```python
from build123d import *

# Parameters (mm, degrees)
SKETCH1_W               = 2000
SKETCH1_H               = 420
SKETCH1_W_2             = 1782.939992392
SKETCH1_H_2             = 340
BOSS_EXTRUDE1_DEPTH     = 20
SKETCH3_W               = 30
SKETCH3_H               = 80
BOSS_EXTRUDE2_DEPTH     = 200
FILLET1_R               = 40
FILLET2_R               = 40
SKETCH5_W               = 972.378142936
SKETCH5_H               = 20.021799472
SKETCH5_W_2             = 1944.756285872
BOSS_EXTRUDE5_DEPTH     = 20
CUT_EXTRUDE3_DEPTH      = 2088
CUT_EXTRUDE3_DEPTH_BACK = 85
SKETCH9_R               = 28.284271247


with BuildPart() as part:
    # Sketch1 → Boss-Extrude1 (new body)
    with BuildSketch(Plane(origin=(0, 0, 0), x_dir=(1, 0, 0), z_dir=(0, 1, 0))):
        Rectangle(SKETCH1_W, SKETCH1_H)
        Rectangle(SKETCH1_W_2, SKETCH1_H_2, mode=Mode.SUBTRACT)
    extrude(amount=BOSS_EXTRUDE1_DEPTH)

    # Sketch3 → Boss-Extrude2 (add)
    with BuildSketch(Plane(origin=(0, 20, 0), x_dir=(1, 0, 0), z_dir=(0, 1, 0))):
        with Locations((-985, 170)):
            Rectangle(SKETCH3_W, SKETCH3_H)
        with Locations((985, -170)):
            Rectangle(SKETCH3_W, SKETCH3_H)
        with Locations((985, 170)):
            Rectangle(SKETCH3_W, SKETCH3_H)
        with Locations((-985, -170)):
            Rectangle(SKETCH3_W, SKETCH3_H)
    extrude(amount=BOSS_EXTRUDE2_DEPTH)

    # Fillet1
    fillet1_edges = [part.edges().sort_by_distance(p)[0] for p in [
        (-985, 220, -210),
        (-985, 220, -130),
        (-985, 220, 130),
        (-985, 220, 210),
        (985, 220, -210),
        (985, 220, -130),
        (985, 220, 130),
        (985, 220, 210),
    ]]
    fillet(fillet1_edges, radius=FILLET1_R - 0.0001)  # a hair under: the kernel refuses the full size

    # Fillet2
    fillet2_edges = [part.edges().sort_by_distance(p)[0] for p in [
        (985, 20, 130),
        (985, 20, -130),
        (-985, 20, -130),
        (-985, 20, 130),
    ]]
    fillet(fillet2_edges, radius=FILLET2_R)

    # Sketch5 → Boss-Extrude5 (add)
    with BuildSketch(Plane(origin=(0, 20, 0), x_dir=(1, 0, 0), z_dir=(0, 1, 0))):
        with Locations((486.189071468, -190)):
            Rectangle(SKETCH5_W, SKETCH5_H)
        with Locations((0, 190)):
            Rectangle(SKETCH5_W_2, SKETCH5_H)
        with Locations((-486.189071468, -190)):
            Rectangle(SKETCH5_W, SKETCH5_H)
    extrude(amount=BOSS_EXTRUDE5_DEPTH)

    # Sketch9 → Cut-Extrude3 (cut, two sides: drawn at the far end of the back side and taken through both)
    with BuildSketch(Plane.ZY.offset(-970).offset(-CUT_EXTRUDE3_DEPTH_BACK)):
        with Locations(Location((-170, 180, 0), (0, 0, 180))):
            Circle(SKETCH9_R)
        with Locations(Location((170, 180, 0), (0, 0, 180))):
            Circle(SKETCH9_R)
    extrude(amount=CUT_EXTRUDE3_DEPTH + CUT_EXTRUDE3_DEPTH_BACK, mode=Mode.SUBTRACT)


solid = part.part
```
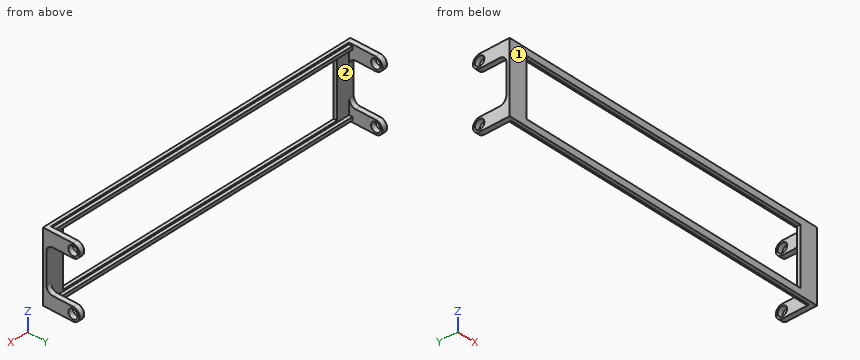
Could you check a few things on this model? Use its own coordinates, in mm. Face numbers are marked on the shaded views. Round coordinates to 2 decimals unless told otherwise and drop trailing zeros. Loops run counter-clockwise (first coordinate to the right, second up) from the corner with the lowest first, then second, coordinate; pieces in that order, holes last. Notation, with made-up numbers: M -16,1 L 38,1 A19 ccw 38,32 Z; hole C -14.5,87 d8. An arc over 180 degrees is marked long. Write item = value, one per line.
1. I need wall thicknesses on probe 1 along Z at (x, y) = (461.5, 39.5); probe 2 along Y at (x, z) = (-978, 170); probe 3 along X at (y, z) = (104.5, -159). Which ranges of each line are inside material? Lowest first, please.
Results below:
probe_1 = -200.01 to -179.99, 179.99 to 200.01
probe_2 = 0 to 151.72, 208.28 to 220
probe_3 = -1000 to -970, 970 to 1000
2. I want a section at B-B, the plane z = -3. Write out the boundary of the cut face in (x, y).
Results below:
outline = M -1000,0 L -891.47,0 L -891.47,20 L -1000,20 Z; M 891.47,0 L 1000,0 L 1000,20 L 891.47,20 Z
3. Will these pins go through, and if not, where does the flat tip stop? P1, Ø8, axis at x = -198.5, z = -207, coming from the +Y side; P2, Ø10, axis at x = 396, y = 35, coming from the +Z side.
Results below:
P1 = 20
P2 = 200.01
4. I want a section at C-C, the plane x = -115. Write out the boundary of the cut face in (y, z), and give its area (3 significant figures).
Results below:
outline = M 0,-210 L 20,-210 L 20,-200.01 L 40,-200.01 L 40,-179.99 L 20,-179.99 L 20,-170 L 0,-170 Z; M 0,170 L 20,170 L 20,179.99 L 40,179.99 L 40,200.01 L 20,200.01 L 20,210 L 0,210 Z
area = 2,400 mm²
5. I want a section at A-A, the plane y = 96. Write out the boundary of the cut face in (x, z), and give its area (3 significant figures).
Results below:
outline = M -1000,-210 L -970,-210 L -970,-130 L -1000,-130 Z; M -1000,130 L -970,130 L -970,210 L -1000,210 Z; M 970,-210 L 1000,-210 L 1000,-130 L 970,-130 Z; M 970,130 L 1000,130 L 1000,210 L 970,210 Z
area = 9,600 mm²
6. Thinking about a two-plate mould opening in X: for the marked faces 1 and 2, which applies, +X half, -X half, draft (parallel to the pull), parting line (faces both ways), or undercut?
Results below:
face_1 = draft
face_2 = undercut
